CAD build for the part. Positions are in the model's coordinates, mm. A direction names the side the tool comes from. Coordinates: 2 decimals unless noted, no trailing zeros. Order: outer loops, then holes, each group sorted by start corner. A loop starts at its lowest first (then second) coordinate and runs counter-clockwise, first axis right, second up. Notation, with made-up numbers: (-27, 45) - (-7, 45) arc R28 ccw to (-7, 71) - close; hole circle Ø4 at (83, -36). An arc over 180 degrees is marked (long way). Write each question's results on one line, items separated by ' | '. Start each with the question number.
Q1. Band-saw the part on B-B, the plane z = 234.5. Write the cut outline in (x, y).
Q2. Wall check: probe 1 along Z at (x, y) = (150, -7.5); probe 2 along X at (y, z) = (-3.5, 131); probe 3 along X at (y, z) = (-7.75, 132.5). Give the ranges that are in metal, low to high.
Q3. Pull direction X, two halves, no side cores. Call faces 6 (the flat face through (148, 0, 213)), 7 (the flat face through (10, -5, 360)), 8 (the flat face through (70.075, -5, 415)): released by +X, released by -X, zero draft, split by the parting line, or undercut.
Q4. Which spindle directions (+Z, -Z, +X, -X, +Y, -Y) get a long thin tool onto all of the face, cutting with end or side? Do faces 1 (the flat face through (290, -5, 120)), 2 (the flat face through (240, -5, 5)), 3 (the flat face through (100, -5, 420)), 4 (the flat face through (5, -5, 130)), 5 (the flat face through (295, -5, 390.075)). Say none if no direction does.
Q5. Band-saw the part on A-A, the plane z = 85. Write the cut outline in (x, y).
Q6. Pin check, flat tips, straight feed: P1, Ø4, axis at x = 170.5, y = -6.5, coming from the -Z side; P2, Ø1.5, axis at y = -7.5, z = 112.5, coming from the +X side; P3, Ø5, axis at x = 4.5, y = -5, coming from the -Z side; P4, Ø3, axis at y = -3.5, z = 6.5, coming from the -X side. Stop position of each tip, or through.
```python
from build123d import *

# Parameters (mm, degrees)
F0_W     = 300
F0_H     = 420
F1_DEPTH = 10
F2_W     = 10
F2_H     = 10
F2_W_2   = 19.925
F2_H_2   = 19.925
F3_DEPTH = 10.001
F4_R     = 60
F5_DEPTH = 10.001


with BuildPart() as f1:
    # F0 (on Front) → F1 (new body)
    with BuildSketch(Plane.XZ):
        with Locations((150, 210)):
            Rectangle(F0_W, F0_H)
    extrude(amount=F1_DEPTH)

    # F2 (on face) → F3 (cut, through all)
    with BuildSketch(Plane(origin=(0, 0, 0), x_dir=(-1, 0, 0), z_dir=(0, 1, 0))):
        with Locations((-295, 5)):
            Rectangle(F2_W, F2_H)
        with Locations((-270.0375, 5)):
            Rectangle(F2_W_2, F2_H)
        with Locations((-230.0375, 5)):
            Rectangle(F2_W_2, F2_H)
        with Locations((-190.0375, 5)):
            Rectangle(F2_W_2, F2_H)
        with Locations((-150.0375, 5)):
            Rectangle(F2_W_2, F2_H)
        with Locations((-110.0375, 5)):
            Rectangle(F2_W_2, F2_H)
        with Locations((-70.0375, 5)):
            Rectangle(F2_W_2, F2_H)
        with Locations((-30.0375, 5)):
            Rectangle(F2_W_2, F2_H)
        with Locations((-5, 5)):
            Rectangle(F2_W, F2_H)
        with Locations((-295, 40.0375)):
            Rectangle(F2_W, F2_H_2)
        with Locations((-295, 80.0375)):
            Rectangle(F2_W, F2_H_2)
        with Locations((-295, 120.0375)):
            Rectangle(F2_W, F2_H_2)
        with Locations((-295, 160.0375)):
            Rectangle(F2_W, F2_H_2)
        with Locations((-295, 200.0375)):
            Rectangle(F2_W, F2_H_2)
        with Locations((-295, 240.0375)):
            Rectangle(F2_W, F2_H_2)
        with Locations((-295, 280.0375)):
            Rectangle(F2_W, F2_H_2)
        with Locations((-295, 320.0375)):
            Rectangle(F2_W, F2_H_2)
        with Locations((-295, 360.0375)):
            Rectangle(F2_W, F2_H_2)
        with Locations((-295, 400.0375)):
            Rectangle(F2_W, F2_H_2)
        with Locations((-295, 415)):
            Rectangle(F2_W, F2_H)
        with Locations((-280.0375, 415)):
            Rectangle(F2_W_2, F2_H)
        with Locations((-240.0375, 415)):
            Rectangle(F2_W_2, F2_H)
        with Locations((-200.0375, 415)):
            Rectangle(F2_W_2, F2_H)
        with Locations((-160.0375, 415)):
            Rectangle(F2_W_2, F2_H)
        with Locations((-120.0375, 415)):
            Rectangle(F2_W_2, F2_H)
        with Locations((-80.0375, 415)):
            Rectangle(F2_W_2, F2_H)
        with Locations((-40.0375, 415)):
            Rectangle(F2_W_2, F2_H)
        Polygon((9.925, 420), (-10, 420), (-10, 410), (0, 410), (9.925, 410), align=None)
        with Locations((-5, 400.0375)):
            Rectangle(F2_W, F2_H_2)
        with Locations((-5, 360.0375)):
            Rectangle(F2_W, F2_H_2)
        with Locations((-5, 320.0375)):
            Rectangle(F2_W, F2_H_2)
        with Locations((-5, 280.0375)):
            Rectangle(F2_W, F2_H_2)
        with Locations((-5, 240.0375)):
            Rectangle(F2_W, F2_H_2)
        with Locations((-5, 200.0375)):
            Rectangle(F2_W, F2_H_2)
        with Locations((-5, 160.0375)):
            Rectangle(F2_W, F2_H_2)
        with Locations((-5, 120.0375)):
            Rectangle(F2_W, F2_H_2)
        with Locations((-5, 80.0375)):
            Rectangle(F2_W, F2_H_2)
        with Locations((-5, 40.0375)):
            Rectangle(F2_W, F2_H_2)
    extrude(amount=-F3_DEPTH, mode=Mode.SUBTRACT)

    # F4 (on face) → F5 (cut, through all)
    with BuildSketch(Plane(origin=(0, 0, 0), x_dir=(-1, 0, 0), z_dir=(0, 1, 0))):
        with Locations((-150, 130)):
            Circle(F4_R)
    extrude(amount=-F5_DEPTH, mode=Mode.SUBTRACT)


solid = f1.part
```
Results below:
1) outline: (10, -10) - (290, -10) - (290, 0) - (10, 0) - close
2) probe 1: z = 10 to 70, 190 to 420 | probe 2: x = 0 to 90.01, 209.99 to 300 | probe 3: x = 0 to 90.05, 209.95 to 300
3) face 6: zero draft | face 7: released by -X | face 8: undercut
4) face 1: +X, +Y, -Y | face 2: -Z, +Y, -Y | face 3: +Z, +X, -X, +Y, -Y | face 4: -X, +Y, -Y | face 5: +Z, +X, +Y, -Y
5) outline: (10, -10) - (110.31, -10) - (110.31, 0) - (10, 0) - close; (189.69, -10) - (290, -10) - (290, 0) - (189.69, 0) - close
6) P1: stops at z = 0 | P2: stops at x = 290 | P3: stops at z = 10 | P4: stops at x = 10
